Geometry check sheet. Reference: the model listing, model coordinates, mm. A direction names the side the tool comes from. Round coordinates to 2 decimals unless told otherwise and drop trailing zeros. Order: outer loops, then holes, each group sorted by start corner. A loop starts at its lowest first (then second) coordinate and runs counter-clockwise, first axis right, second up.
(1) Thickness scan on L1, parallel to X at y = 134, z = 0.75; L2, parallel to X at y = 89, z = 1.5. Record the ranges inside material, lowest first.
(2) Draft check along Y on faces 4 (the face through (96.1, 45.9, 6)), 5 (the face through (140, 69, 1)), 6 (the face through (139, 138, 2)). Enter one of: pulls with the +Y half, pulls with the -Y half, needs draft (parallel to the pull), parting line crosses it, or undercut.
(3) Gauge pin test, flat end, axial feed: P1, Ø5, axis at x = 99.5, y = 81.5, coming from the +Z side. Record the tip position at first contact, or that the pin passes through.
(4) Cross-section at C-C on y = 17. Enter the section's corners in (x, z).
(5) Set-up check for faces 1 (the face through (128, 20, 2)), 2 (the face through (94.67, 102.52, 4.48)), 3 (the face through (0, 71, 1)): record each of +Z, -Z, +X, -X, +Y, -Y from which the full face is reachable in a straight line by a thin tool's end or side.
(6) Cross-section at A-A on x = 31. Enter the section's corners in (y, z).
Autodesk Inventor part; units mm, degrees
ref_plane "YZ Plane" through (0, 0, 0) normal (1, 0, 0) x (0, 1, 0)
ref_plane "XZ Plane" through (0, 0, 0) normal (0, 1, 0) x (-1, 0, 0)
ref_plane "XY Plane" through (0, 0, 0) normal (0, 0, 1) x (1, 0, 0)
sketch "Sketch1" plane through (0, 0, 0) normal (0, 0, 1) x (1, 0, 0)
  line L0 (0, 0) -> (140, 0)
  line L1 (140, 0) -> (140, 140)
  line L2 (140, 140) -> (0, 140)
  line L3 (0, 140) -> (0, 0)
  dimension "d0" = 140
  dimension "d1" = 140
extrude "Extrusion1" add sketch "Sketch1" along normal blind 3
fillet "Fillet1" radius 5 4 edges at (140, 140, 1.5) (140, 0, 1.5) (0, 140, 1.5) (0, 0, 1.5)
sketch "Sketch4" plane through (0, 0, 3) normal (0, 0, 1) x (1, 0, 0)
  line L0 (135, 140) -> (5, 140)
  line L1 (0, 135) -> (0, 5)
  line L2 (140, 5) -> (140, 135)
  line L3 (5, 0) -> (135, 0)
  point P0 (0, 0)
  point P1 (6, 134)
  point P2 (134, 134)
  point P3 (6, 6)
  point P4 (134, 6)
  dimension "d30" = 6
  dimension "d31" = 6
  dimension "d32" = 6
  dimension "d33" = 6
  dimension "d34" = 6
  dimension "d35" = 6
  dimension "d36" = 6
  dimension "d37" = 6
hole "Hole2" at (134, 134, 3) at (6, 6, 3) at (134, 6, 3) at (6, 134, 3) direction (0, 0, -1) diameter 4 depth 15
sketch "Sketch5" plane through (0, 0, 3) normal (0, 0, 1) x (1, 0, 0)
  line L0 (20, 130) -> (120, 130)
  line L1 (120, 130) -> (120, 125)
  line L2 (120, 125) -> (20, 125)
  line L3 (20, 125) -> (20, 130)
  line L4 (135, 140) -> (5, 140)
  line L5 (140, 5) -> (140, 135)
  line L6 (20, 15) -> (120, 15)
  line L7 (120, 15) -> (120, 10)
  line L8 (120, 10) -> (20, 10)
  line L9 (20, 10) -> (20, 15)
  line L10 (5, 0) -> (135, 0)
  line L11 (10, 120) -> (15, 120)
  line L12 (15, 120) -> (15, 20)
  line L13 (15, 20) -> (10, 20)
  line L14 (10, 20) -> (10, 120)
  line L15 (0, 135) -> (0, 5)
  line L16 (125, 120) -> (130, 120)
  line L17 (130, 120) -> (130, 20)
  line L18 (130, 20) -> (125, 20)
  line L19 (125, 20) -> (125, 120)
  point P0 (0, 0)
  dimension "d45" = 10
  dimension "d46" = 5
  dimension "d47" = 20
  dimension "d48" = 100
  dimension "d49" = 100
  dimension "d50" = 5
  dimension "d51" = 20
  dimension "d52" = 10
  dimension "d53" = 5
  dimension "d54" = 100
  dimension "d55" = 20
  dimension "d56" = 10
  dimension "d57" = 5
  dimension "d58" = 100
  dimension "d59" = 10
  dimension "d60" = 20
extrude "Extrusion4" cut sketch "Sketch5" against normal blind 10
sketch "Sketch6" plane through (0, 0, 3) normal (0, 0, 1) x (1, 0, 0)
  circle A0 centre (46, 105) radius 2.5
  circle A1 centre (95, 105) radius 2.5
  circle A2 centre (46, 47) radius 2.5
  circle A3 centre (95, 47) radius 2.5
  line L0 (140, 5) -> (140, 135)
  line L1 (135, 140) -> (5, 140)
  point P0 (0, 0)
  dimension "d66" = 5
  dimension "d67" = 5
  dimension "d68" = 5
  dimension "d69" = 5
  dimension "d70" = 58
  dimension "d71" = 58
  dimension "d72" = 49
  dimension "d73" = 0
  dimension "d74" = 45
  dimension "d76" = 49
  dimension "d77" = 35
  dimension "d79" = 0
extrude "Extrusion5" add sketch "Sketch6" along normal blind 3
sketch "Sketch7" plane through (46, 105, 6) normal (0, 0, 1) x (1, 0, 0)
  circle A0 centre (0, 0) radius 1.35
  circle A1 centre (49, 0) radius 2.5
  circle A2 centre (49, 0) radius 1.35
  circle A3 centre (49, -58) radius 2.5
  circle A4 centre (49, -58) radius 1.35
  circle A5 centre (0, -58) radius 1.35
  point P0 (-46, -105)
  point P1 (49, -55.5)
  dimension "d82" = 2.7
  dimension "d83" = 2.7
  dimension "d84" = 2.7
  dimension "d85" = 2.7
extrude "Extrusion6" add sketch "Sketch7" along normal blind 3 contours A0 | A2 | A4 | A5
properties part number "Led deksel niet hub"
Found:
1. L1: x = 0 to 4, 8 to 132, 136 to 140
1. L2: x = 0 to 10, 15 to 125, 130 to 140
2. face 4: undercut
2. face 5: needs draft
2. face 6: pulls with the +Y half
3. P1: stops at z = 3
4. outline: (0, 0) - (140, 0) - (140, 3) - (0, 3) - close
5. face 1: +Z, -Z
5. face 2: +Z
5. face 3: +Z, -Z, -X, +Y, -Y
6. outline: (0, 0) - (10, 0) - (10, 3) - (0, 3) - close; (15, 0) - (125, 0) - (125, 3) - (15, 3) - close; (130, 0) - (140, 0) - (140, 3) - (130, 3) - close
